Can you work these out from the model? Positions are in its coordinate system, mm. Face numbers are marked on the shaded views. Give positions to 0.01 mm unless a question says otherwise; leave off trailing zeros. Order: outer loops, then holes, each group sorted by start corner. A loop starts at its lowest first (then second) coordinate and runs counter-clockwise, first axis right, second up.
```python
from build123d import *

# Parameters (mm, degrees)
SKETCH1_W           = 60
SKETCH1_H           = 65
SKETCH1_R           = 2.625
SKETCH1_R_2         = 2.1
BOSS_EXTRUDE1_DEPTH = 6.35
FILLET1_R           = 10
SKETCH2_R           = 4
CUT_EXTRUDE1_DEPTH  = 7.35


with BuildPart() as part:
    # Sketch1 → Boss-Extrude1 (new body)
    with BuildSketch(Plane(origin=(0, 0, 0), x_dir=(1, 0, 0), z_dir=(0, 1, 0))):
        with Locations((30, -32.5)):
            Rectangle(SKETCH1_W, SKETCH1_H)
        with Locations((10, -10)):
            Circle(SKETCH1_R, mode=Mode.SUBTRACT)
        with Locations((30, -10)):
            Circle(SKETCH1_R, mode=Mode.SUBTRACT)
        with Locations((50, -10)):
            Circle(SKETCH1_R, mode=Mode.SUBTRACT)
        with Locations((22.27, -30)):
            Circle(SKETCH1_R_2, mode=Mode.SUBTRACT)
        with Locations((35, -55)):
            Circle(SKETCH1_R_2, mode=Mode.SUBTRACT)
    extrude(amount=BOSS_EXTRUDE1_DEPTH)

    # Fillet1
    fillet1_edges = [part.edges().sort_by_distance(p)[0] for p in [
        (60, 3.175, 65),
    ]]
    fillet(fillet1_edges, radius=FILLET1_R)

    # Sketch2 → Cut-Extrude1 (cut, through all)
    with BuildSketch(Plane(origin=(0, 6.35, 0), x_dir=(1, 0, 0), z_dir=(0, 1, 0))):
        with Locations((50, -30)):
            Circle(SKETCH2_R)
        with Locations((50, -50)):
            Circle(SKETCH2_R)
    extrude(amount=-CUT_EXTRUDE1_DEPTH, mode=Mode.SUBTRACT)


solid = part.part
```
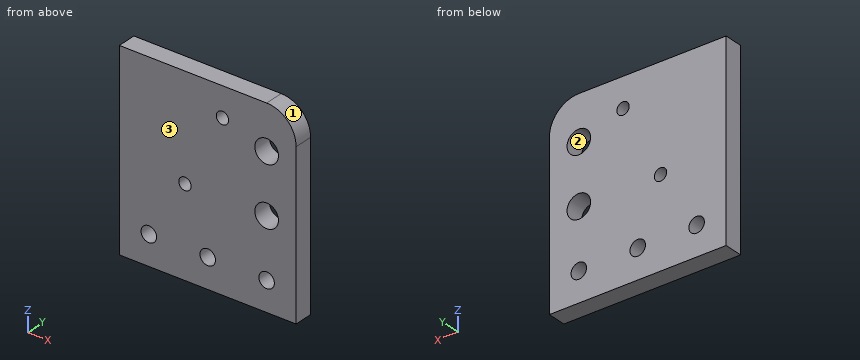
1) Suppose I cut it at D-D (z = 10). Please give me the cut outline in (x, y) (3 decimals), and give its area (3 significant figures).
2) Suppose I cut it at B-B (x = 35). Please give me the cut outline in (y, z).
3) Suppose I cut it at A-A (z = 30). Please give me the cut outline in (x, y).
4) If I drill on line 1 (X direction, y = 2.75, z = 10) (3 decimals); line 2 (X direction, y = 1.5, z = 30); line 3 (Z direction, x = 53, y = 4.5), over which ranges is the centre line in solid material (lowest first)?
5) I'm going to push flat-ended pins straight in: pin 1 Ø6.5 at (x, z) = (50, 30) entering from -Y; pin 2 Ø8.5 at (x, z) = (10, 10) entering from -Y. Where does each tip first touch, or does it pass through?
6) Suppose I cut it at C-C (y = 2.25). Please give me the cut outline in (x, z) (3 decimals), and give its area (3 significant figures).
7) We'd pull the mould along Z, two halves only. Please class the marked faces 1, 2 and 3: +Z half, -Z half, draft (parallel to the pull), parting line (faces both ways), or undercut.
Results:
1. outline: (0, 0) - (7.375, 0) - (7.375, 6.35) - (0, 6.35) - close; (12.625, 0) - (27.375, 0) - (27.375, 6.35) - (12.625, 6.35) - close; (32.625, 0) - (47.375, 0) - (47.375, 6.35) - (32.625, 6.35) - close; (52.625, 0) - (60, 0) - (60, 6.35) - (52.625, 6.35) - close
1. area: 281 mm2
2. outline: (0, 0) - (6.35, 0) - (6.35, 52.9) - (0, 52.9) - close; (0, 57.1) - (6.35, 57.1) - (6.35, 65) - (0, 65) - close
3. outline: (0, 0) - (20.17, 0) - (20.17, 6.35) - (0, 6.35) - close; (24.37, 0) - (46, 0) - (46, 6.35) - (24.37, 6.35) - close; (54, 0) - (60, 0) - (60, 6.35) - (54, 6.35) - close
4. line 1: x = 0 to 7.375, 12.625 to 27.375, 32.625 to 47.375, 52.625 to 60
4. line 2: x = 0 to 20.17, 24.37 to 46, 54 to 60
4. line 3: z = 0 to 27.35, 32.65 to 47.35, 52.65 to 64.54
5. pin 1: passes through
5. pin 2: stops at y = 0
6. outline: (0, 0) - (60, 0) - (60, 55) arc R10 ccw to (50, 65) - (0, 65) - close; hole circle Ø5.25 at (10, 10); hole circle Ø4.2 at (22.27, 30); hole circle Ø5.25 at (30, 10); hole circle Ø4.2 at (35, 55); hole circle Ø8 at (50, 30); hole circle Ø8 at (50, 50); hole circle Ø5.25 at (50, 10)
6. area: 3,690 mm2
7. face 1: +Z half
7. face 2: undercut
7. face 3: draft
